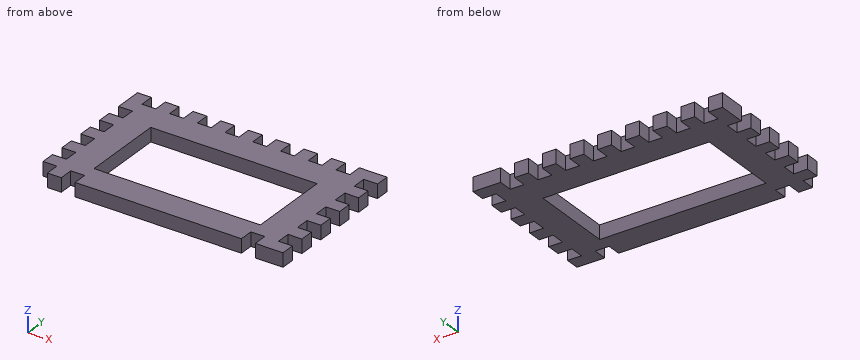
Autodesk Inventor part; units mm, degrees
ref_plane "YZ Plane" through (0, 0, 0) normal (1, 0, 0) x (0, 1, 0)
ref_plane "XZ Plane" through (0, 0, 0) normal (0, 1, 0) x (-1, 0, 0)
ref_plane "XY Plane" through (0, 0, 0) normal (0, 0, 1) x (1, 0, 0)
sketch "Sketch1" plane through (0, 0, 0) normal (0, 0, 1) x (1, 0, 0)
  line L0 (5, 5) -> (85, 5)
  line L1 (85, 5) -> (85, 55)
  line L2 (85, 55) -> (5, 55)
  line L3 (5, 55) -> (5, 5)
  line L4 (0, 60) -> (5, 60)
  line L5 (5, 60) -> (5, 55)
  line L6 (5, 55) -> (0, 55)
  line L7 (0, 55) -> (0, 60)
  line L8 (0, 50) -> (5, 50)
  line L9 (5, 50) -> (5, 55)
  line L10 (5, 55) -> (0, 55)
  line L11 (0, 55) -> (0, 50)
  line L12 (5, 45) -> (0, 45)
  line L13 (0, 40) -> (5, 40)
  line L14 (5, 40) -> (5, 45)
  line L15 (5, 45) -> (0, 45)
  line L16 (0, 45) -> (0, 40)
  line L17 (5, 35) -> (0, 35)
  line L18 (0, 30) -> (5, 30)
  line L19 (5, 30) -> (5, 35)
  line L20 (5, 35) -> (0, 35)
  line L21 (0, 35) -> (0, 30)
  line L22 (5, 25) -> (0, 25)
  line L23 (0, 20) -> (5, 20)
  line L24 (5, 20) -> (5, 25)
  line L25 (5, 25) -> (0, 25)
  line L26 (0, 25) -> (0, 20)
  line L27 (5, 15) -> (0, 15)
  line L28 (0, 10) -> (5, 10)
  line L29 (5, 10) -> (5, 15)
  line L30 (5, 15) -> (0, 15)
  line L31 (0, 15) -> (0, 10)
  line L32 (15, 55) -> (10, 55)
  line L33 (15, 55) -> (10, 55)
  line L34 (10, 60) -> (15, 60)
  line L35 (10, 55) -> (10, 60)
  line L36 (15, 60) -> (15, 55)
  line L37 (25, 55) -> (20, 55)
  line L38 (25, 55) -> (20, 55)
  line L39 (20, 60) -> (25, 60)
  line L40 (20, 55) -> (20, 60)
  line L41 (25, 60) -> (25, 55)
  line L42 (35, 55) -> (30, 55)
  line L43 (35, 55) -> (30, 55)
  line L44 (30, 60) -> (35, 60)
  line L45 (30, 55) -> (30, 60)
  line L46 (35, 60) -> (35, 55)
  line L47 (45, 55) -> (40, 55)
  line L48 (45, 55) -> (40, 55)
  line L49 (40, 60) -> (45, 60)
  line L50 (40, 55) -> (40, 60)
  line L51 (45, 60) -> (45, 55)
  line L52 (55, 55) -> (50, 55)
  line L53 (55, 55) -> (50, 55)
  line L54 (50, 60) -> (55, 60)
  line L55 (50, 55) -> (50, 60)
  line L56 (55, 60) -> (55, 55)
  line L57 (65, 55) -> (60, 55)
  line L58 (65, 55) -> (60, 55)
  line L59 (60, 60) -> (65, 60)
  line L60 (60, 55) -> (60, 60)
  line L61 (65, 60) -> (65, 55)
  line L62 (75, 55) -> (70, 55)
  line L63 (75, 55) -> (70, 55)
  line L64 (70, 60) -> (75, 60)
  line L65 (70, 55) -> (70, 60)
  line L66 (75, 60) -> (75, 55)
  line L67 (85, 55) -> (80, 55)
  line L68 (85, 55) -> (80, 55)
  line L69 (80, 60) -> (85, 60)
  line L70 (80, 55) -> (80, 60)
  line L71 (85, 60) -> (85, 55)
  line L72 (90, 60) -> (85, 60)
  line L73 (85, 60) -> (85, 55)
  line L74 (85, 55) -> (90, 55)
  line L75 (90, 55) -> (90, 60)
  line L76 (90, 50) -> (85, 50)
  line L77 (85, 45) -> (90, 45)
  line L78 (90, 45) -> (90, 50)
  line L79 (90, 40) -> (85, 40)
  line L80 (85, 35) -> (90, 35)
  line L81 (90, 35) -> (90, 40)
  line L82 (90, 30) -> (85, 30)
  line L83 (85, 25) -> (90, 25)
  line L84 (90, 25) -> (90, 30)
  line L85 (90, 20) -> (85, 20)
  line L86 (85, 15) -> (90, 15)
  line L87 (90, 15) -> (90, 20)
  line L88 (90, 10) -> (85, 10)
  line L89 (85, 5) -> (90, 5)
  line L90 (90, 5) -> (90, 10)
  line L91 (10, 10) -> (15, 10)
  line L92 (15, 10) -> (15, 5)
  line L93 (15, 5) -> (10, 5)
  line L94 (10, 5) -> (10, 10)
  line L95 (75, 10) -> (80, 10)
  line L96 (80, 10) -> (80, 5)
  line L97 (80, 5) -> (75, 5)
  line L98 (75, 5) -> (75, 10)
  line L99 (15, 45) -> (75, 45)
  line L100 (75, 45) -> (75, 15)
  line L101 (75, 15) -> (15, 15)
  line L102 (15, 15) -> (15, 45)
  point P0 (0, 0)
  point P1 (10, 50)
  point P2 (20, 50)
  point P3 (30, 50)
  point P4 (40, 50)
  point P5 (50, 50)
  point P6 (60, 50)
  point P7 (70, 50)
  point P8 (80, 50)
  dimension "d2" = 10
  dimension "d9" = 10
  dimension "d16" = 10
extrude "Extrusion1" add sketch "Sketch1" along normal blind 5 contours L3 L2 L1 L0 L96 L95 L98 L92 L91 L94 | L28 L31 L27 L3 | L23 L26 L22 L3 | L1 L88 L90 L89 | L18 L21 L17 L3 | L1 L85 L87 L86 | L13 L16 L12 L3 | L1 L82 L84 L83 | L8 L11 L6 L3 | L6 L7 L4 L5 | L1 L79 L81 L80 | L35 L34 L36 L2 | L1 L76 L78 L77 | L40 L39 L41 L2 | L2 L70 L69 L71 | L71 L72 L75 L74 | L45 L44 L46 L2 | L2 L65 L64 L66 | L50 L49 L51 L2 | L2 L60 L59 L61 | L55 L54 L56 L2
properties part number "leftrightsidehole"
Source: CAD feature listing. Evaluate the final solid. Frame: model axes, mm. Give positions to 0.01 mm unless a question says otherwise; leave off trailing zeros. Loops run counter-clockwise (first coordinate to the right, second up) from the corner with the lowest first, then second, coordinate; pieces in that order, holes last. Notation, with made-up numbers: (84.25, -9.5) -> (111.25, -9.5) arc R34 cw to (111.25, 23.5) -> close; hole circle Ø5 at (63.25, -32). An arc over 180 degrees is marked (long way). Use a Markdown table: item, result. Add a question column.
(1) First-contact query: pin 1 Ø2.5 at (y, z) = (32.5, 2) entering from +X; pin 2 Ø2.5 at (y, z) = (38, 2) entering from -X; pin 3 Ø2.5 at (x, z) = (57.5, 1.5) entering from +Y. Flat tips, straight axial feed; report the tip coordinate or a pass-through.
(2) Ray query, line 1 (X direction, y = 9.5, z = 4.1); line 2 (Y direction, x = 49, z = 1.4); line 3 (X direction, y = 27.5, z = 2.95). Return the intervals inside material, ascending.
(3) Section query A-A (y = 34). Output: boundary loops of the cut face in (x, z).
(4) Section query B-B (y = 11.5). Output: boundary loops of the cut face in (x, z), then the cut area to 3 significant figures.
Checked values:
| question | item | result |
|---|---|---|
| 1 | pin 1 | x = 85 |
| 1 | pin 2 | x = 5 |
| 1 | pin 3 | y = 55 |
| 2 | line 1 | 5 to 10, 15 to 75, 80 to 90 |
| 2 | line 2 | 5 to 15, 45 to 55 |
| 2 | line 3 | 5 to 15, 75 to 90 |
| 3 | outline | (0, 0) -> (15, 0) -> (15, 5) -> (0, 5) -> close; (75, 0) -> (85, 0) -> (85, 5) -> (75, 5) -> close |
| 4 | outline | (0, 0) -> (85, 0) -> (85, 5) -> (0, 5) -> close |
| 4 | area | 425 mm^2 |
